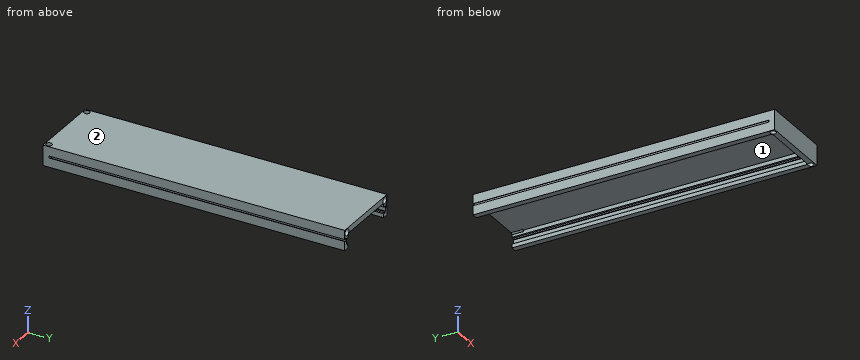
```python
from build123d import *

# Parameters (mm, degrees)
P_IDAT_VYSUNUT_M2_DEPTH        = 3
P_IDAT_VYSUNUT_M2_DEPTH_BACK   = 4.5
SKICA1_W                       = 2
SKICA1_H                       = 153.5
P_IDAT_VYSUNUT_M2_2_DEPTH      = 3
P_IDAT_VYSUNUT_M2_2_DEPTH_BACK = 4.5
SKICA3_W                       = 2
SKICA3_H                       = 153.5
P_IDAT_VYSUNUT_M3_DEPTH        = 1
SKICA5_W                       = 0.5
SKICA5_H                       = 0.3
SKICA5_H_2                     = 1.5
ODEBRAT_VYSUNUT_M2_DEPTH       = 158.729198312
SKICA6_W                       = 1
SKICA6_H                       = 2
P_IDAT_VYSUNUT_M4_DEPTH        = 153.5
SKICA7_W                       = 38
SKICA7_H                       = 153.5
P_IDAT_VYSUNUT_M5_DEPTH        = 3
SKICA8_W                       = 38
SKICA8_H                       = 10.5
P_IDAT_VYSUNUT_M6_DEPTH        = 3
SKICA4_W                       = 0.5
SKICA4_H                       = 0.3
SKICA4_H_2                     = 1.5
ODEBRAT_VYSUNUT_M3_DEPTH       = 158.779117756
ODEBRAT_VYSUNUT_M6_DEPTH       = 153.5
ODEBRAT_START                  = -10.5
SKICA14_R                      = 1.5
ODEBRAT_VYSUNUT_M9_DEPTH       = 10.5
SKICA22_R                      = 2
SKICA22_R_2                    = 1.5
P_IDAT_VYSUNUT_M12_DEPTH       = 10.5
P_IDAT_START                   = -7.5
SKICA15_R                      = 2
SKICA15_R_2                    = 1.75
P_IDAT_VYSUNUT_M7_DEPTH        = 7.5
SKICA16_R                      = 1.75
ODEBRAT_VYSUNUT_M10_DEPTH      = 4
SKICA17_R                      = 2
SKICA17_R_2                    = 1.75
P_IDAT_VYSUNUT_M10_DEPTH       = 4
P_IDAT_VYSUNUT_M11_DEPTH       = 2


with BuildPart() as part:
    # Skica1 → P_idat vysunut_m2 (new, two sides: drawn at the far end of the back side and taken through both)
    with BuildSketch(Plane.XY.offset(-P_IDAT_VYSUNUT_M2_DEPTH_BACK)):
        with Locations((1, 74.75)):
            Rectangle(SKICA1_W, SKICA1_H)
    extrude(amount=P_IDAT_VYSUNUT_M2_DEPTH + P_IDAT_VYSUNUT_M2_DEPTH_BACK)

    # Skica3 → P_idat vysunut_m3 (add)
    with BuildSketch(Plane.ZY):
        with Locations((-3.5, 74.75)):
            Rectangle(SKICA3_W, SKICA3_H)
        with Locations((2, 74.75)):
            Rectangle(SKICA3_W, SKICA3_H)
    extrude(amount=P_IDAT_VYSUNUT_M3_DEPTH)



with BuildPart() as body_2:
    # Skica1 → P_idat vysunut_m2 2 (new, two sides: drawn at the far end of the back side and taken through both)
    with BuildSketch(Plane.XY.offset(-P_IDAT_VYSUNUT_M2_2_DEPTH_BACK)):
        with Locations((-35, 74.75)):
            Rectangle(SKICA1_W, SKICA1_H)
    extrude(amount=P_IDAT_VYSUNUT_M2_2_DEPTH + P_IDAT_VYSUNUT_M2_2_DEPTH_BACK)

    # Skica5 → Odebrat vysunut_m2 (cut, through all)
    with BuildSketch(Plane.XZ.offset(2)):
        with Locations((-34.25, -1.65)):
            Rectangle(SKICA5_W, SKICA5_H)
        with Locations((-34.25, -0.75)):
            Rectangle(SKICA5_W, SKICA5_H_2)
        with Locations((-34.25, 0.15)):
            Rectangle(SKICA5_W, SKICA5_H)
    extrude(amount=-ODEBRAT_VYSUNUT_M2_DEPTH, mode=Mode.SUBTRACT)

    # Skica6 → P_idat vysunut_m4 (add, through all)
    with BuildSketch(Plane.XZ.offset(2)):
        with Locations((-33.5, 2)):
            Rectangle(SKICA6_W, SKICA6_H)
        with Locations((-33.5, -3.5)):
            Rectangle(SKICA6_W, SKICA6_H)
    extrude(amount=-P_IDAT_VYSUNUT_M4_DEPTH)


with BuildPart() as part_1:
    add(part.part)

    add(body_2.part)  # P_idat vysunut_m5 merges body 2
    # Skica7 → P_idat vysunut_m5 (add)
    with BuildSketch(Plane.XY.offset(3)):
        with Locations((-17, 74.75)):
            Rectangle(SKICA7_W, SKICA7_H)
    extrude(amount=P_IDAT_VYSUNUT_M5_DEPTH)

    # Skica8 → P_idat vysunut_m6 (add)
    with BuildSketch(Plane.XZ.offset(2)):
        with Locations((-17, 0.75)):
            Rectangle(SKICA8_W, SKICA8_H)
    extrude(amount=P_IDAT_VYSUNUT_M6_DEPTH)

    # Skica4 → Odebrat vysunut_m3 (cut, through all)
    with BuildSketch(Plane.XZ.offset(2)):
        with Locations((0.25, 0.15)):
            Rectangle(SKICA4_W, SKICA4_H)
        with Locations((0.25, -0.75)):
            Rectangle(SKICA4_W, SKICA4_H_2)
        with Locations((0.25, -1.65)):
            Rectangle(SKICA4_W, SKICA4_H)
    extrude(amount=-ODEBRAT_VYSUNUT_M3_DEPTH, mode=Mode.SUBTRACT)

    # Skica11 → Odebrat vysunut_m6 (cut)
    with BuildSketch(Plane(origin=(-33, -2, 3), x_dir=(1, 0, 0), z_dir=(0, -1, 0))):
        Polygon((-2, -1.25), (-2, -3.25), (-3, -2.75), (-3, -1.75), align=None)
        Polygon((34, -1.25), (35, -1.75), (35, -2.75), (34, -3.25), align=None)
    extrude(amount=-ODEBRAT_VYSUNUT_M6_DEPTH, mode=Mode.SUBTRACT)

    # Skica14 → Odebrat vysunut_m9 (cut)
    with BuildSketch(Plane(origin=(0, 0, -4.5), x_dir=(-1, 0, 0), z_dir=(0, 0, -1)).offset(ODEBRAT_START)):
        with Locations((34, -3)):
            Circle(SKICA14_R)
        with Locations(Location((0, -3, 0), (0, 0, 41.810314896))):
            Circle(SKICA14_R)
    extrude(amount=ODEBRAT_VYSUNUT_M9_DEPTH, mode=Mode.SUBTRACT)

    # Skica22 → P_idat vysunut_m12 (add)
    # profile 1 of 2: a face of its own
    with BuildSketch(Plane.XY.offset(6)):
        with Locations((-34, -3)):
            Circle(SKICA22_R)
        with Locations(Location((-34, -3, 0), (0, 0, 180))):
            Circle(SKICA22_R_2, mode=Mode.SUBTRACT)
    # profile 2 of 2: a face of its own
    with BuildSketch(Plane.XY.offset(6)):
        with Locations((0, -3)):
            Circle(SKICA22_R)
        with Locations((0, -3)):
            Circle(SKICA22_R_2, mode=Mode.SUBTRACT)
    extrude(amount=-P_IDAT_VYSUNUT_M12_DEPTH)

    # Skica15 → P_idat vysunut_m7 (add)
    # profile 1 of 2: a face of its own
    with BuildSketch(Plane(origin=(0, 0, -4.5), x_dir=(-1, 0, 0), z_dir=(0, 0, -1)).offset(P_IDAT_START)):
        with Locations((34, -3)):
            Circle(SKICA15_R)
        with Locations((34, -3)):
            Circle(SKICA15_R_2, mode=Mode.SUBTRACT)
    # profile 2 of 2: a face of its own
    with BuildSketch(Plane(origin=(0, 0, -4.5), x_dir=(-1, 0, 0), z_dir=(0, 0, -1)).offset(P_IDAT_START)):
        with Locations((0, -3)):
            Circle(SKICA15_R)
        with Locations((0, -3)):
            Circle(SKICA15_R_2, mode=Mode.SUBTRACT)
    extrude(amount=P_IDAT_VYSUNUT_M7_DEPTH)

    # Skica16 → Odebrat vysunut_m10 (cut)
    with BuildSketch(Plane(origin=(0, 151.5, 0), x_dir=(1, 0, 0), z_dir=(0, 1, 0))):
        with Locations((0, -4)):
            Circle(SKICA16_R)
        with Locations((-34, -4)):
            Circle(SKICA16_R)
    extrude(amount=-ODEBRAT_VYSUNUT_M10_DEPTH, mode=Mode.SUBTRACT)

    # Skica17 → P_idat vysunut_m10 (add)
    # profile 1 of 2: a face of its own
    with BuildSketch(Plane(origin=(0, 151.5, 0), x_dir=(1, 0, 0), z_dir=(0, 1, 0))):
        with Locations((0, -4)):
            Circle(SKICA17_R)
        with Locations(Location((0, -4, 0), (0, 0, 270))):
            Circle(SKICA17_R_2, mode=Mode.SUBTRACT)
    # profile 2 of 2: a face of its own
    with BuildSketch(Plane(origin=(0, 151.5, 0), x_dir=(1, 0, 0), z_dir=(0, 1, 0))):
        with Locations((-34, -4)):
            Circle(SKICA17_R)
        with Locations(Location((-34, -4, 0), (0, 0, 34.849904579))):
            Circle(SKICA17_R_2, mode=Mode.SUBTRACT)
    extrude(amount=-P_IDAT_VYSUNUT_M10_DEPTH)

    # Skica18 → P_idat vysunut_m11 (add)
    with BuildSketch(Plane.XZ.offset(-147.5)):
        with BuildLine():
            Line((-33, 2.267949192), (-33, 3))
            Line((-33, 3), (-32.267949192, 3))
            ThreePointArc((-32.267949192, 3), (-32.48236191, 2.48236191), (-33, 2.267949192))
        make_face()
        with BuildLine():
            Line((-1.732050808, 3), (-1, 3))
            Line((-1, 3), (-1, 2.267949192))
            ThreePointArc((-1, 2.267949192), (-1.51763809, 2.48236191), (-1.732050808, 3))
        make_face()
    extrude(amount=P_IDAT_VYSUNUT_M11_DEPTH)


solid = part_1.part
```
CAD build for the part. Positions are in the model's coordinates, mm. Face numbers are marked on the shaded views. Coordinates: 2 decimals unless noted, no trailing zeros. Order: outer loops, then holes, each group sorted by start corner. A loop starts at its lowest first (then second) coordinate and runs counter-clockwise, first axis right, second up. Notation, with made-up numbers: (53.5, -17.5) - (87.5, -17.5) arc R17 cw to (87.5, 15.5) - close; hole circle Ø11 at (-4, 25.25). An arc over 180 degrees is marked (long way). Answer in a Markdown table with one row per item.
1. Pull direction X, two halves, no side cores. Call the marked faces 1 and 2: +X half, -X half, draft (parallel to the pull), parting line (faces both ways), or undercut.
Answer:
| item | result |
|---|---|
| face 1 | undercut |
| face 2 | draft |
2. Drill centre lines: L1, parallel to X at y = 12, z = 2.75; L2, parallel to X at y = 149.25, z = 4; L3, parallel to Y at x = -9, z = -0.75. Where is each one in solid material? Low to high. Write a range as from..to.
Answer:
| item | result |
|---|---|
| L1 | -36..-33, -1..2 |
| L2 | -36..-35.75, -32.25..-1.75, 1.75..2 |
| L3 | -5..-2 |
3. Slice it at B-B, the plane x = -19.5. List the corners of the cut face in (y, z).
Answer:
| item | result |
|---|---|
| outline | (-5, -4.5) - (-2, -4.5) - (-2, 3) - (151.5, 3) - (151.5, 6) - (-5, 6) - close |
4. Flat gauge pin, fed straight in: P1, Ø12, axis at x = -25, y = 120.5, coming from the -Z side. Where does the tip first touch, or does it go through?
Answer:
| item | result |
|---|---|
| P1 | z = 3 |
